Verification items for this drawing (mm, ordinates from the low corner). A direction names the side the tool comes from. Give positions to 0.01 mm unless a question says otherwise; leave off trailing zeros. Write each loop counter-clockwise with the first axis right and the second up, starting at its lowest first coordinate (ties: lowest second). Pieces come first, ordered by that corner, then holes. Notation, with made-up numbers: (75.5, -27.5) -> (110.5, -27.5) arc R22 cw to (110.5, -14.5) -> close; hole circle Ø7 at (32.25, 83.5). An arc over 180 degrees is marked (long way). Answer as a JSON object with one key per item and string values.
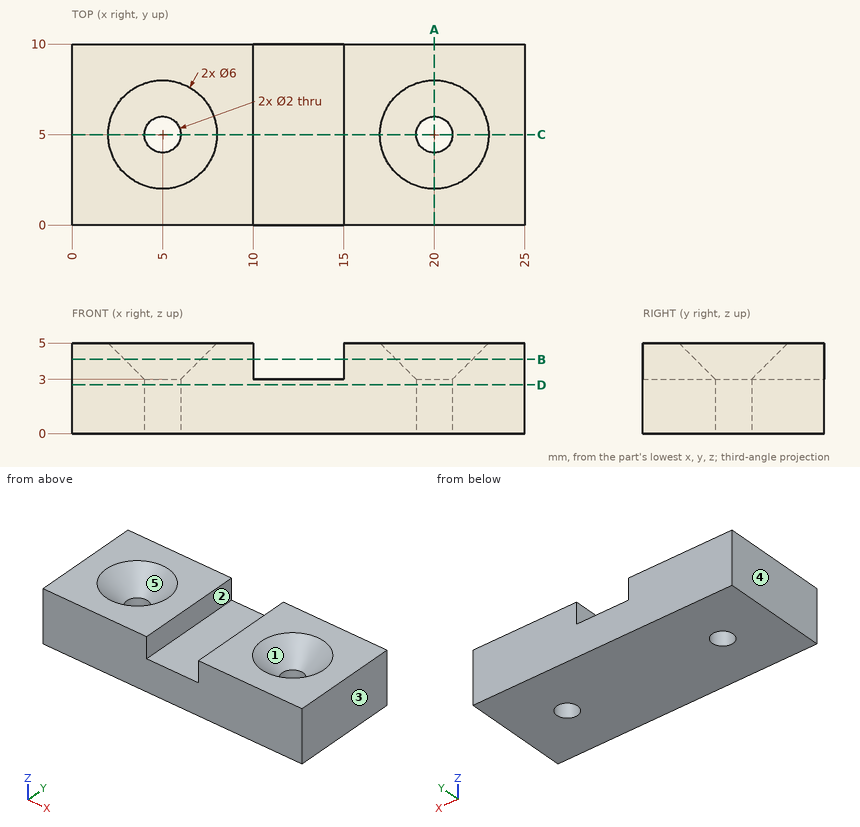
1. Sectioned sample at D-D, the plane z = 2.7. Enter the section's corners in (x, y).
Determined:
{"outline": "(0, 0) -> (25, 0) -> (25, 10) -> (0, 10) -> close; hole circle Ø2 at (5, 5); hole circle Ø2 at (20, 5)"}
2. Mould release check, pull along X, two halves, no side actions. Record for the marked faces 3, 4 and 5: released by +X, released by -X, zero draft, split by the parting line, or undercut.
Determined:
{"face 3": "released by +X", "face 4": "released by -X", "face 5": "undercut"}
3. Sectioned sample at C-C, the plane y = 5. Enter the section's corners in (x, z), plus the area to 3 significant figures.
Determined:
{"outline": "(0, 0) -> (4, 0) -> (4, 3) -> (2, 5) -> (0, 5) -> close; (6, 0) -> (19, 0) -> (19, 3) -> (17, 5) -> (15, 5) -> (15, 3) -> (10, 3) -> (10, 5) -> (8, 5) -> (6, 3) -> close; (21, 0) -> (25, 0) -> (25, 5) -> (23, 5) -> (21, 3) -> close", "area": "87.0 mm^2"}
4. Go/stop test with flat-tipped pins: P1, Ø3, axis at x = 5, y = 5, coming from the +Z side; P2, Ø4, axis at x = 12.5, y = 5, coming from the +Z side. Record where each tip stops, or that it passes through.
Determined:
{"P1": "z = 3.5", "P2": "z = 3"}
5. Scan lines: L1, parallel to X at y = 5, z = 0.7; L2, parallel to X at y = 3.75, z = 3.9; L3, parallel to Y at x = 20, z = 1.4. Record each from-to range of solid material in increasing order. Write a range as [from, to].
Determined:
{"L1": "[0, 4], [6, 19], [21, 25]", "L2": "[0, 3.57], [6.43, 10], [15, 18.57], [21.43, 25]", "L3": "[0, 4], [6, 10]"}
6. Access from +Z, -Z, +X, -X, +Y, -Y to the whole of each face (thin tool, end or side, straight path). Record for the marked faces 1 and 2.
Determined:
{"face 1": "+Z", "face 2": "+Z, +Y, -Y"}
7. Sectioned sample at B-B, the plane z = 4.1. Enter the section's corners in (x, y).
Determined:
{"outline": "(0, 0) -> (10, 0) -> (10, 10) -> (0, 10) -> close; (15, 0) -> (25, 0) -> (25, 10) -> (15, 10) -> close; hole circle Ø4.2 at (5, 5); hole circle Ø4.2 at (20, 5)"}
8. Sectioned sample at A-A, the plane x = 20. Enter the section's corners in (y, z), plus the area to 3 significant figures.
Determined:
{"outline": "(0, 0) -> (4, 0) -> (4, 3) -> (2, 5) -> (0, 5) -> close; (6, 0) -> (10, 0) -> (10, 5) -> (8, 5) -> (6, 3) -> close", "area": "36.0 mm^2"}
